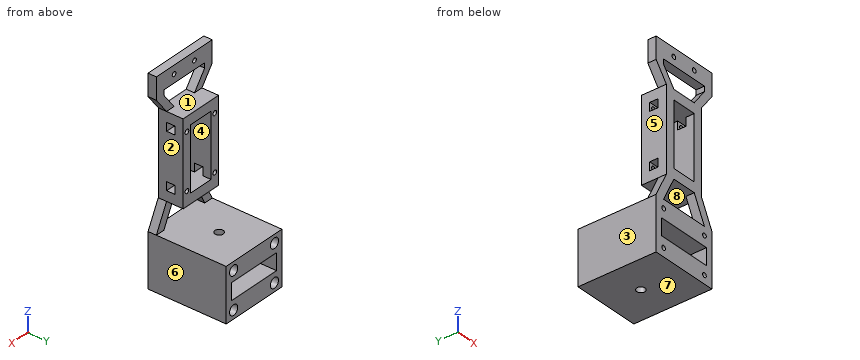
Autodesk Inventor part; units mm, degrees
ref_plane "YZ Plane" through (0, 0, 0) normal (1, 0, 0) x (0, 1, 0)
ref_plane "XZ Plane" through (0, 0, 0) normal (0, 1, 0) x (-1, 0, 0)
ref_plane "XY Plane" through (0, 0, 0) normal (0, 0, 1) x (1, 0, 0)
sketch "Sketch1" plane through (0, 0, 0) normal (0, 1, 0) x (-1, 0, 0)
  line L0 (20.5, -60) -> (-20.5, -60)
  line L1 (-20.5, -60) -> (-20.5, 60)
  line L2 (-20.5, 60) -> (20.5, 60)
  line L3 (20.5, -60) -> (-20.5, 60) construction
  line L4 (-20.5, -60) -> (20.5, 60) construction
  circle A0 centre (7.5, 55) radius 1.35
  circle A1 centre (-7.5, 55) radius 1.35
  circle A2 centre (15, -33) radius 1.35
  circle A3 centre (15, -55) radius 1.35
  circle A4 centre (-15, -55) radius 1.35
  circle A5 centre (-15, -33) radius 1.35
  line L5 (-13, -13) -> (-13, 37)
  line L6 (13, 37) -> (13, -13)
  line L7 (20.5, -33) -> (20.5, -28)
  line L8 (20.5, -28) -> (13, -13)
  line L9 (-13, -13) -> (-20.5, -28)
  line L10 (20.5, 55) -> (20.5, 54)
  line L11 (20.5, 47) -> (13, 37)
  line L12 (-13, 37) -> (-20.5, 47)
  line L13 (20.5, 60) -> (20.5, 47)
  line L14 (20.5, -28) -> (20.5, -60)
  line L15 (16.5, -49) -> (-16.5, -49)
  line L16 (-16.5, -49) -> (-16.5, -39)
  line L17 (-16.5, -39) -> (16.5, -39)
  line L18 (16.5, -39) -> (16.5, -49)
  line L19 (15, -28) -> (-15, -28)
  line L20 (-15, -28) -> (-7.5, -13)
  line L21 (-7.5, -13) -> (7.5, -13)
  line L22 (7.5, -13) -> (15, -28)
  line L23 (7.5, -7) -> (-7.5, -7)
  line L24 (-7.5, -7) -> (-7.5, 31)
  line L25 (-7.5, 31) -> (7.5, 31)
  line L26 (7.5, 31) -> (7.5, -7)
  line L27 (7.5, 37) -> (-7.5, 37)
  line L28 (-7.5, 37) -> (-15, 47)
  line L29 (7.5, 37) -> (15, 47)
  line L30 (15, 47) -> (15, 50)
  line L31 (15, 50) -> (-15, 50)
  line L32 (-15, 50) -> (-15, 47)
  point P0 (0, 0)
  dimension "d0" = 41
  dimension "d1" = 120
  dimension "d2" = 5
  dimension "d3" = 2.7
  dimension "d5" = 22
  dimension "d6" = 15
  dimension "d7" = 7.5
  dimension "d8" = 30
  dimension "d9" = 15
  dimension "d10" = 88
  dimension "d11" = 50
  dimension "d12" = 26
  dimension "d14" = 13
  dimension "d15" = 5
  dimension "d16" = 8
  dimension "d17" = 33
  dimension "d18" = 16.5
  dimension "d19" = 10
  dimension "d20" = 6
  dimension "d21" = 5
  dimension "d22" = 15
  dimension "d23" = 6
  dimension "d25" = 6
  dimension "d28" = 5.5
  dimension "d29" = 5.5
  dimension "d30" = 5
  dimension "d33" = 0
  dimension "d34" = 5.5
  dimension "d35" = 5.5
extrude "Extrusion1" add sketch "Sketch1" along normal blind 5 contours L0 L1 L9 L5 L12 L2 L13 L10 L11 L6 L8 L7 L14
sketch "Sketch2" plane through (0, 5, 0) normal (0, 1, 0) x (1, 0, 0)
  line L0 (-20.5, 60) -> (-20.5, 28)
  line L1 (-7.5, 13) -> (-15, 28)
  line L2 (-20.5, 28) -> (-15, 28)
  line L3 (15, 28) -> (7.5, 13)
  line L4 (13, 13) -> (20.5, 28)
  line L5 (15, 28) -> (20.5, 28)
  line L6 (20.5, 60) -> (-20.5, 60)
  line L7 (20.5, 28) -> (20.5, 60)
  line L8 (16.5, 39) -> (-16.5, 39)
  line L9 (-15, 28) -> (15, 28)
  circle A0 centre (-15, 33) radius 1.35
  circle A1 centre (15, 33) radius 1.35
  line L10 (-16.5, 49) -> (16.5, 49)
  line L11 (-16.5, 39) -> (-16.5, 49)
  line L12 (16.5, 49) -> (16.5, 39)
  circle A2 centre (15, 55) radius 1.35
  circle A3 centre (-15, 55) radius 1.35
  circle A4 centre (-15, 55) radius 3
  circle A5 centre (15, 55) radius 3
  circle A6 centre (15, 33) radius 3
  circle A7 centre (-15, 33) radius 3
  point P0 (0, 0)
  dimension "d36" = 6
  dimension "d37" = 6
  dimension "d38" = 6
  dimension "d39" = 6
extrude "Extrusion2" add sketch "Sketch2" along normal blind 42 contours L6 L7 L5 L9 L2 L0
sketch "Sketch3" plane through (-15, 0, -28) normal (0, 0, 1) x (1, 0, 0)
  line L0 (-5.5, 5) -> (-5.5, 47)
  line L1 (-5.5, 47) -> (35.5, 47)
  point P0 (15, 0)
  point P1 (15, 26)
  dimension "d42" = 20.5
  dimension "d43" = 21
hole "Hole1" at (0, 26, -28) direction (0, 0, -1) diameter 5 end through all
sketch "Sketch4" plane through (0, 5, 0) normal (0, 1, 0) x (1, 0, 0)
  line L0 (-7.5, -31) -> (-7.5, 7)
  line L1 (7.5, 7) -> (7.5, -31)
  line L2 (-7.5, 7) -> (7.5, 7)
  line L3 (7.5, -31) -> (-7.5, -31)
  line L4 (13, -37) -> (13, 13)
  line L5 (-13, 13) -> (13, 13)
  line L6 (13, 13) -> (13, -37)
  line L7 (13, -37) -> (-13, -37)
  line L8 (-13, -37) -> (-13, 13)
  circle A0 centre (-10.25, 4.5) radius 1.35
  circle A1 centre (-10.25, -28.5) radius 1.35
  circle A2 centre (10.25, -28.5) radius 1.35
  circle A3 centre (10.25, 4.5) radius 1.35
  point P0 (0, 0)
  dimension "d63" = 2.7
  dimension "d64" = 2.5
  dimension "d65" = 2.5
  dimension "d66" = 2.75
  dimension "d67" = 2.75
extrude "Extrusion5" add sketch "Sketch4" along normal blind 10
sketch "Sketch5" plane through (-13, 0, -13) normal (-1, 0, 0) x (0, 0, 1)
  line L0 (0, 0) -> (0, 5) construction
  line L1 (60, 5) -> (50, 5) construction
  line L2 (6, 5) -> (11, 5)
  line L3 (11, 5) -> (11, 10)
  line L4 (11, 10) -> (6, 10)
  line L5 (6, 10) -> (6, 5)
  line L6 (44, 5) -> (39, 5)
  line L7 (39, 5) -> (39, 10)
  line L8 (39, 10) -> (44, 10)
  line L9 (44, 10) -> (44, 5)
  point P0 (13, 0)
  dimension "d53" = 5
  dimension "d54" = 5
  dimension "d55" = 0
  dimension "d56" = 5
  dimension "d57" = 5
  dimension "d58" = 6
  dimension "d59" = 6
  dimension "d60" = 5
extrude "Extrusion4" cut sketch "Sketch5" against normal through all
properties part number "Houder encodere"
Model file for the job. Use its own axes, mm. Face numbers are marked on the shaded views. A direction names the side the tool comes from. Coordinates: 2 decimals unless noted, no trailing zeros. Loops run counter-clockwise (first coordinate to the right, second up) from the corner with the lowest first, then second, coordinate; pieces in that order, holes last. Notation, with made-up numbers: (-21, 78.5) - (-2, 78.5) arc R23 cw to (-2, 112.5) - close; hole circle Ø6 at (-8.75, -27). An arc over 180 degrees is marked (long way). Write item = value, one per line. Start each with the question number.
Item 1: Pull direction Z, two halves, no side cores. Call the marked faces 5, 6, 7 and 8: +Z half, -Z half, draft (parallel to the pull), parting line (faces both ways), or undercut.
Item 2: Saw through at A-A, the plane y = 26. List the corners of the cut face in (x, z), then the cut area to 3 significant figures.
Item 3: Saw through at C-C, the plane z = 1. List the corners of the cut face in (x, y).
Item 4: 3-axis set-ups, long thin cutter, end or side, ignore diameter. For the marked faces 1, 2, 3 and 4: which of +Z, -Z, +X, -X, +Y, -Y reach the whole face in a straight line?
Item 5: Saw through at B-B, the plane z = -33. List the corners of the cut face in (x, y), then the cut area to 3 significant figures.
Item 6: Drop flat-ended pins along their axis: pin 1 Ø5 at (x, z) = (9.5, 46.5) entering from +Y; pin 2 Ø4.5 at (y, z) = (8.5, 2) entering from -X; pin 3 Ø1.5 at (x, z) = (11.5, 28.5) entering from +Y; pin 4 Ø1.8 at (x, z) = (14.5, -55) entering from +Y. Give the stop position or say it passes through.
Item 7: Wall check: probe 1 along Z at (x, y) = (-15, 27); probe 2 along Z at (x, y) = (9, 7); probe 3 along Z at (x, y) = (10, 11). Give the ranges that are in metal, low to high. Write a range as [from, to].
Item 8: Saw through at D-D, the plane y = 6.5. State how many separate pieces and enclosed holes the cut face has, then the cut area to 3 significant figures.
Answers:
q1.face_5 = undercut
q1.face_6 = draft
q1.face_7 = -Z half
q1.face_8 = undercut
q2.outline = (-20.5, -60) - (-2.5, -60) - (-2.5, -49) - (-16.5, -49) - (-16.5, -39) - (-2.5, -39) - (-2.5, -28) - (-20.5, -28) - close; (2.5, -60) - (20.5, -60) - (20.5, -28) - (2.5, -28) - (2.5, -39) - (16.5, -39) - (16.5, -49) - (2.5, -49) - close; hole circle Ø6 at (-15, -55); hole circle Ø6 at (-15, -33); hole circle Ø6 at (15, -55); hole circle Ø6 at (15, -33)
q2.area = 759 mm2
q3.outline = (-13, 0) - (-7.5, 0) - (-7.5, 15) - (-13, 15) - close; (7.5, 0) - (13, 0) - (13, 15) - (7.5, 15) - close
q4.face_1 = +Y
q4.face_2 = +X, +Y, -Y
q4.face_3 = +Z, -Z, -X, +Y, -Y
q4.face_4 = +Y, -Y
q5.outline = (-20.5, 0) - (-16.35, 0) - (-16.35, 5) - (-18, 5) - (-18, 47) - (-20.5, 47) - close; (-13.65, 0) - (13.65, 0) - (13.65, 5) - (12, 5) - (12, 47) - (-12, 47) - (-12, 5) - (-13.65, 5) - close; (16.35, 0) - (20.5, 0) - (20.5, 47) - (18, 47) - (18, 5) - (16.35, 5) - close; hole circle Ø5 at (0, 26)
q5.area = 1,380 mm2
q6.pin_1 = through
q6.pin_2 = -13
q6.pin_3 = 15
q6.pin_4 = 5
q7.probe_1 = [-60, -58], [-52, -49], [-39, -36], [-30, -28]
q7.probe_2 = [-60, -49], [-39, -28], [-13, -7], [-2, 26], [31, 37]
q7.probe_3 = [-60, -49], [-39, -28], [-13, -5.83], [-3.17, 27.17], [29.83, 37]
q8.separate_pieces = 5
q8.enclosed_holes = 5
q8.area = 1,490 mm2
